The model under review builds one solid part; all positions refer to its coordinate system, in mm. Round coordinates to 2 decimals unless told otherwise and drop trailing zeros. Loops run counter-clockwise (first coordinate to the right, second up) from the corner with the lowest first, then second, coordinate; pieces in that order, holes last. Notation, with made-up numbers: (56.5, 16) -> (106.5, 16) arc R22 ccw to (106.5, 43) -> close; hole circle Ø11 at (-4.75, 21). An arc over 180 degrees is marked (long way). Use a Markdown table: item, result. Add a question column.
1) Consider section B-B on x = -64. Give the boundary of the cut face in (y, z).
2) Insertion check: pin 1 (2.5 mm diameter, centred on y = -137, z = 2, fed in from +X); pin 2 (2.5 mm diameter, centred on x = -88, z = 3, fed in from -Y). Each pin has a flat end and moves straight along its axis. Give the tip position at first contact, or say it passes through.
3) Consider section A-A on z = 3.2. Give the boundary of the cut face in (x, y), plus the area to 3 significant figures.
4) Wall thickness on probe 1 along X at (y, z) = (-71, 3); probe 2 along Y at (x, z) = (-65, 4.6): over which ranges is each line inside the solid? List them lowest first.
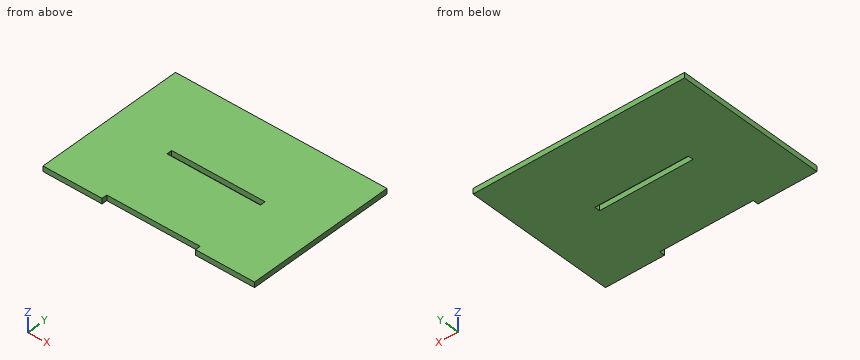
Autodesk Inventor part; units mm, degrees
ref_plane "YZ Plane" through (0, 0, 0) normal (1, 0, 0) x (0, 1, 0)
ref_plane "XZ Plane" through (0, 0, 0) normal (0, 1, 0) x (-1, 0, 0)
ref_plane "XY Plane" through (0, 0, 0) normal (0, 0, 1) x (1, 0, 0)
sketch "Sketch1" plane through (0, 0, 0) normal (0, 0, 1) x (1, 0, 0)
  line L0 (0, 0) -> (-197, 0)
  line L1 (-197, 0) -> (-197, -140)
  line L2 (-197, -140) -> (0, -140)
  line L3 (0, -140) -> (0, 0)
  dimension "d0" = 140
  dimension "d1" = 197
extrude "Extrusion1" add sketch "Sketch1" along normal blind 5
sketch "Sketch3" plane through (0, 0, 5) normal (0, 0, 1) x (1, 0, 0)
  line L0 (0, 0) -> (-197, 0)
  line L1 (0, -140) -> (0, 0)
  line L2 (-197, -140) -> (0, -140)
  line L3 (-197, 0) -> (-197, -140)
  line L4 (-142, -140) -> (-55, -140)
  line L5 (-55, -140) -> (-55, -135)
  line L6 (-55, -135) -> (-142, -135)
  line L7 (-142, -135) -> (-142, -140)
  line L8 (-141, -72.5) -> (-54, -72.5)
  line L9 (-54, -72.5) -> (-54, -67.5)
  line L10 (-54, -67.5) -> (-141, -67.5)
  line L11 (-141, -67.5) -> (-141, -72.5)
  point P0 (-55, -140)
  dimension "d13" = 5
  dimension "d14" = 55
  dimension "d15" = 55
  dimension "d16" = 5
  dimension "d17" = 72.5
extrude "Extrusion3" cut sketch "Sketch3" against normal blind 5 contours L2 L7 L6 L5 | L11 L10 L9 L8
properties part number "Frente"
Result set:
| question | item | result |
|---|---|---|
| 1 | outline | (-135, 0) -> (-72.5, 0) -> (-72.5, 5) -> (-135, 5) -> close; (-67.5, 0) -> (0, 0) -> (0, 5) -> (-67.5, 5) -> close |
| 2 | pin 1 | x = 0 |
| 2 | pin 2 | y = -135 |
| 3 | outline | (-197, -140) -> (-142, -140) -> (-142, -135) -> (-55, -135) -> (-55, -140) -> (0, -140) -> (0, 0) -> (-197, 0) -> close; hole (-141, -72.5) -> (-54, -72.5) -> (-54, -67.5) -> (-141, -67.5) -> close |
| 3 | area | 26,700 mm2 |
| 4 | probe 1 | -197 to -141, -54 to 0 |
| 4 | probe 2 | -135 to -72.5, -67.5 to 0 |
